The listing builds one solid part. Answer for the finished solid, in the listing's coordinates (mm). A direction names the side the tool comes from. Coordinates: 2 decimals unless noted, no trailing zeros. Write each loop counter-clockwise with the first axis right and the second up, starting at its lowest first coordinate (ties: lowest second). Pieces come first, ordered by that corner, then holes. Notation, with made-up numbers: M 47,49 L 65,49 A32 cw 65,87 Z; hole C -32.5,17.25 d3. An arc over 180 degrees is marked long. Answer as CSV lines item,"result".
```python
from build123d import *

# Parameters (mm, degrees)
SKETCH2_R           = 6.35
SKETCH2_R_2         = 3.5
BOSS_EXTRUDE1_DEPTH = 10
BOSS_EXTRUDE2_DEPTH = 10
SKETCH2_4_W         = 10
SKETCH2_4_H         = 15
SKETCH2_4_R         = 1.5
BOSS_EXTRUDE3_DEPTH = 7.75
CHAMFER1_SIZE       = 20
CHAMFER1_SIZE_2     = 11.547005384


with BuildPart() as part:
    # Sketch2 → Boss-Extrude1 (new body)
    with BuildSketch(Plane.XY):
        with BuildLine():
            ThreePointArc((11.35, 0), (0, 11.35), (-11.35, 0))
            Line((-11.35, 0), (-11.35, -30))
            Line((-11.35, -30), (11.35, -30))
            Line((11.35, -30), (11.35, 0))
        make_face()
        Circle(SKETCH2_R, mode=Mode.SUBTRACT)
        with Locations((-0.790227169, -19)):
            Circle(SKETCH2_R_2, mode=Mode.SUBTRACT)
    extrude(amount=BOSS_EXTRUDE1_DEPTH)

    # Sketch2<3> → Boss-Extrude2 (add)
    with BuildSketch(Plane.XY):
        with BuildLine():
            ThreePointArc((11.35, -7.197992776), (0, -13.44), (-11.35, -7.197992776))
            Line((-11.35, -7.197992776), (-11.35, -30))
            Line((-11.35, -30), (-5.790227169, -30))
            Line((-5.790227169, -30), (-5.790227169, -15))
            Line((-5.790227169, -15), (4.209772831, -15))
            Line((4.209772831, -15), (4.209772831, -30))
            Line((4.209772831, -30), (11.35, -30))
            Line((11.35, -30), (11.35, -7.197992776))
        make_face()
    extrude(amount=-BOSS_EXTRUDE2_DEPTH)

    # Sketch2<4> → Boss-Extrude3 (add)
    with BuildSketch(Plane.XY):
        with Locations((-0.790227169, -22.5)):
            Rectangle(SKETCH2_4_W, SKETCH2_4_H)
        with Locations((-0.790227169, -19)):
            Circle(SKETCH2_4_R, mode=Mode.SUBTRACT)
    extrude(amount=-BOSS_EXTRUDE3_DEPTH)

    # Chamfer1
    # the kernel refuses this chamfer: 20, 11.547005384 mm, written as the material it takes off along each edge
    with BuildSketch(Plane(origin=(-63.091715093, -30, 10), x_dir=(0, 0.9998132206222079, 0.019326765612700723), z_dir=(1, 0, 0))) as chamfer1_piece_1:
        Polygon((CHAMFER1_SIZE * 0.999813220622, -CHAMFER1_SIZE * 0.0193267656127), (-CHAMFER1_SIZE_2 * 0.0193267656124, -CHAMFER1_SIZE_2 * 0.999813220604), (0, 0), align=None)
    extrude(amount=126.183430186, mode=Mode.SUBTRACT)

    # Mirror1: part across plane


with BuildPart() as part_1:
    add(part.part)
    add(part.part.mirror(Plane.XY.offset(-10)))


solid = part_1.part
```
Q1. Find section A-A (x = -3). Count the separate pieces of the cut face and the enclosed holes in it, and give its area (3 significant figures).
Output:
separate pieces,"3"
enclosed holes,"0"
area,"582 mm2"
Q2. Flat-ended cylindrical pins translate along their axes: pin 1 Ø1 at (x, z) = (1, -13.5) entering from +Y; pin 2 Ø5 at (x, y) = (1.5, -19.5) entering from +Z; pin 3 Ø1 at (x, z) = (-9, -11.5) entering from +Y. Find the tip coordinate at first contact, or state that the pin passes through.
Output:
pin 1,"y = -13.36"
pin 2,"z = 5.91"
pin 3,"y = -9.51"
Q3. The mould has two halves that part along X. Classify faces 1 (the flat face through (-11.35, -15, -10)), 2 (the flat face through (0, -30, -14)), 3 (the flat face through (-1, -22, -12.25)), 4 (the cylindrical face through (-0.985, -17.513, -3.821)): pulls with the +X half, pulls with the -X half, needs draft (parallel to the pull), parting line crosses it, or undercut.
Output:
face 1,"pulls with the -X half"
face 2,"needs draft"
face 3,"undercut"
face 4,"undercut"
Q4. Find section C-C (z = -11.5). Give the vertices of the cut face in (x, y).
Output:
outline,"M -11.35,-30 L -5.79,-30 L -5.79,-15 L 4.21,-15 L 4.21,-30 L 11.35,-30 L 11.35,-7.2 A13.44 cw -11.35,-7.2 Z"
Q5. Find section D-D (y = -26). Give the vertices of the cut face in (x, z), and give its area (3 significant figures).
Output:
outline,"M -11.35,-20.76 L 11.35,-20.76 L 11.35,0.76 L -11.35,0.76 Z; hole M -5.79,-12.25 L 4.21,-12.25 L 4.21,-7.75 L -5.79,-7.75 Z"
area,"444 mm2"
Q6. Find section B-B (y = -20). Give the vertices of the cut face in (x, z).
Output:
outline,"M -11.35,-24.23 L -4.14,-24.23 L -4.14,-20 L -1.91,-20 L -1.91,-12.25 L -5.79,-12.25 L -5.79,-7.75 L -1.91,-7.75 L -1.91,0 L -4.14,0 L -4.14,4.23 L -11.35,4.23 Z; M 0.33,-20 L 2.56,-20 L 2.56,-24.23 L 11.35,-24.23 L 11.35,4.23 L 2.56,4.23 L 2.56,0 L 0.33,0 L 0.33,-7.75 L 4.21,-7.75 L 4.21,-12.25 L 0.33,-12.25 Z"
Q7. Straight lines are drawn through the part: line 1 (X direction, y = -27.5, z = -8); line 2 (Z direction, x = 10, y = 1); line 3 (Y direction, x = 0, z = -22.5). For each, find the intervals that lie inside material, in ascending order.
Output:
line 1,"-11.35 to -5.79, 4.21 to 11.35"
line 2,"-30 to -20, 0 to 10"
line 3,"-22.99 to -22.41, -15.59 to -6.35, 6.35 to 11.35"
Q8. For faces 5 (the cylindrical face through (0.19, -13.44, -10.14)), 6 (the cylindrical face through (-1.25, -15.53, -22.62)), 7 (the cylindrical face through (-1.25, -15.53, 2.62)), 8 (the cylindrical face through (0.25, 11.347, 4.93)), 9 (the flat face through (4.21, -22, -10)), determine the directions among +Z, -Z, +X, -X, +Y, -Y from which every point of the face is accessible in a straight line to the end or side of a thin tool.
Output:
face 5,"+Y"
face 6,"-Z"
face 7,"+Z"
face 8,"+Z, -Z, +Y"
face 9,"-Y"
